Check sheet for the modelled part. Datum: model origin and axes. Units: mm. A direction names the side the tool comes from. Coordinates: 2 decimals unless noted, no trailing zeros. Loops run counter-clockwise (first coordinate to the right, second up) from the corner with the lowest first, then second, coordinate; pieces in that order, holes last.
```python
from build123d import *

# Parameters (mm, degrees)
SKETCH1_R                = 47.5
BOSS_EXTRUDE1_DEPTH      = 6
BOSS_EXTRUDE1_DEPTH_BACK = 6
SKETCH2_R                = 45
BOSS_EXTRUDE2_DEPTH      = 1
SKETCH3_R                = 45
BOSS_EXTRUDE3_DEPTH      = 1
SKETCH4_R                = 9
BOSS_EXTRUDE4_DEPTH      = 0.2
SKETCH5_R                = 9
BOSS_EXTRUDE5_DEPTH      = 5
SKETCH6_R                = 41
SKETCH6_R_2              = 9
CUT_EXTRUDE1_DEPTH       = 3
SKETCH7_R                = 41
SKETCH7_R_2              = 9
CUT_EXTRUDE2_DEPTH       = 3
SKETCH8_R                = 9
CUT_EXTRUDE3_DEPTH       = 17
SKETCH9_R                = 4
CUT_EXTRUDE4_DEPTH       = 20.2
CUT_EXTRUDE5_REACH       = 58.5
SKETCH10_R               = 1.6
CUT_EXTRUDE6_REACH       = 58.5
SKETCH11_R               = 1.6


with BuildPart() as part:
    # Sketch1 → Boss-Extrude1 (new body, two sides)
    with BuildSketch(Plane.XY) as boss_extrude1_sk:
        Circle(SKETCH1_R)
    extrude(amount=BOSS_EXTRUDE1_DEPTH)
    extrude(boss_extrude1_sk.sketch, amount=-BOSS_EXTRUDE1_DEPTH_BACK)

    # Sketch2 → Boss-Extrude2 (add)
    with BuildSketch(Plane.XY.offset(6)):
        Circle(SKETCH2_R)
    extrude(amount=BOSS_EXTRUDE2_DEPTH)

    # Sketch3 → Boss-Extrude3 (add)
    with BuildSketch(Plane(origin=(0, 0, -6), x_dir=(-1, 0, 0), z_dir=(0, 0, -1))):
        Circle(SKETCH3_R)
    extrude(amount=BOSS_EXTRUDE3_DEPTH)

    # Sketch4 → Boss-Extrude4 (add)
    with BuildSketch(Plane(origin=(0, 0, -7), x_dir=(-1, 0, 0), z_dir=(0, 0, -1))):
        Circle(SKETCH4_R)
    extrude(amount=BOSS_EXTRUDE4_DEPTH)

    # Sketch5 → Boss-Extrude5 (add)
    with BuildSketch(Plane.XY.offset(7)):
        Circle(SKETCH5_R)
    extrude(amount=BOSS_EXTRUDE5_DEPTH)

    # Sketch6 → Cut-Extrude1 (cut)
    with BuildSketch(Plane.XY.offset(7)):
        Circle(SKETCH6_R)
        Circle(SKETCH6_R_2, mode=Mode.SUBTRACT)
    extrude(amount=-CUT_EXTRUDE1_DEPTH, mode=Mode.SUBTRACT)

    # Sketch7 → Cut-Extrude2 (cut)
    with BuildSketch(Plane(origin=(0, 0, -7), x_dir=(-1, 0, 0), z_dir=(0, 0, -1))):
        Circle(SKETCH7_R)
        Circle(SKETCH7_R_2, mode=Mode.SUBTRACT)
    extrude(amount=-CUT_EXTRUDE2_DEPTH, mode=Mode.SUBTRACT)

    # Sketch8 → Cut-Extrude3 (cut, through all)
    with BuildSketch(Plane(origin=(0, 0, -4), x_dir=(-1, 0, 0), z_dir=(0, 0, -1))):
        with Locations((0, 25)):
            Circle(SKETCH8_R)
        with Locations((23.776412907, 7.725424859)):
            Circle(SKETCH8_R)
        with Locations((14.694631307, -20.225424859)):
            Circle(SKETCH8_R)
        with Locations((-14.694631307, -20.225424859)):
            Circle(SKETCH8_R)
        with Locations((-23.776412907, 7.725424859)):
            Circle(SKETCH8_R)
    extrude(amount=-CUT_EXTRUDE3_DEPTH, mode=Mode.SUBTRACT)

    # Sketch9 → Cut-Extrude4 (cut, through all)
    with BuildSketch(Plane.XY.offset(12)):
        Circle(SKETCH9_R)
    extrude(amount=-CUT_EXTRUDE4_DEPTH, mode=Mode.SUBTRACT)

    # Sketch10 → Cut-Extrude5 (cut, up to next)
    with BuildSketch(Plane.ZY.offset(9), mode=Mode.PRIVATE) as cut_extrude5_sk1:
        with Locations((8, 0)):
            Circle(SKETCH10_R)
    cut_extrude5_tool1 = extrude(cut_extrude5_sk1.sketch, amount=-CUT_EXTRUDE5_REACH, mode=Mode.PRIVATE) & part.part
    add(cut_extrude5_tool1.solids().sort_by_distance((-9, 0, 8))[0], mode=Mode.SUBTRACT)

    # Sketch11 → Cut-Extrude6 (cut, up to next)
    with BuildSketch(Plane(origin=(0, 9, 0), x_dir=(1, 0, 0), z_dir=(0, 1, 0)), mode=Mode.PRIVATE) as cut_extrude6_sk1:
        with Locations((0, -8)):
            Circle(SKETCH11_R)
    cut_extrude6_tool1 = extrude(cut_extrude6_sk1.sketch, amount=-CUT_EXTRUDE6_REACH, mode=Mode.PRIVATE) & part.part
    add(cut_extrude6_tool1.solids().sort_by_distance((0, 9, 8))[0], mode=Mode.SUBTRACT)


solid = part.part
```
1) Set-up check for faces 1 (the cylindrical face through (8.314, -3.447, 8.056)), 2 (the flat face through (-4, -2, -7.2)), 3 (the cylindrical face through (1.172, 8.923, -5.622)), 4 (the cylindrical face through (-0.35, 6.37, 9.56)), 5 (the cylindrical face through (1.846, -3.549, 2.534)): record each of +Z, -Z, +X, -X, +Y, -Y from which the full face is reachable in a straight line by a thin tool's end or side.
Answer sheet:
face 1: +Z
face 2: -Z, +X, -X, +Y, -Y
face 3: -Z
face 4: none
face 5: +Z, -Z
2) Section check B-B on y = 25. Enter the section's corners in (x, z), plus the area to 3 significant figures.
Answer sheet:
outline: (-40.39, -6) - (-37.42, -6) - (-37.42, -7) - (-32.5, -7) - (-32.5, -4) - (-9, -4) - (-9, 4) - (-32.5, 4) - (-32.5, 7) - (-37.42, 7) - (-37.42, 6) - (-40.39, 6) - close; (9, -4) - (32.5, -4) - (32.5, -7) - (37.42, -7) - (37.42, -6) - (40.39, -6) - (40.39, 6) - (37.42, 6) - (37.42, 7) - (32.5, 7) - (32.5, 4) - (9, 4) - close
area: 585 mm2
3) Section check D-D on y = 0. Give the number of separate pieces and of enclosed holes in the cut face, plus the area to 3 significant figures.
Answer sheet:
separate pieces: 5
enclosed holes: 0
area: 712 mm2
4) Section check C-C on z = -1.75. Enter the section's corners in (x, y).
Answer sheet:
outline: circle Ø95 at (0, 0); hole circle Ø18 at (-23.78, 7.73); hole circle Ø18 at (-14.69, -20.23); hole circle Ø18 at (0, 25); hole circle Ø8 at (0, 0); hole circle Ø18 at (14.69, -20.23); hole circle Ø18 at (23.78, 7.73)
5) Section check A-A on x = 21.5. Enter the section's corners in (y, z), plus the area to 3 significant figures.
Answer sheet:
outline: (-42.36, -6) - (-39.53, -6) - (-39.53, -7) - (-34.91, -7) - (-34.91, -4) - (-26.11, -4) - (-26.11, 4) - (-34.91, 4) - (-34.91, 7) - (-39.53, 7) - (-39.53, 6) - (-42.36, 6) - close; (-14.34, -4) - (-0.98, -4) - (-0.98, 4) - (-14.34, 4) - close; (16.43, -4) - (34.91, -4) - (34.91, -7) - (39.53, -7) - (39.53, -6) - (42.36, -6) - (42.36, 6) - (39.53, 6) - (39.53, 7) - (34.91, 7) - (34.91, 4) - (16.43, 4) - close
area: 522 mm2
6) Mould release check, pull along Z, two halves, no side actions. Record for faces 6 (the cylindrical face through (-6.37, 0.07, 6.4)), 7 (the flat face through (-10, -40, 7)), 8 (the cylindrical face through (6.11, -17.52, -0.06)): +Z half, -Z half, draft (parallel to the pull), parting line (faces both ways), or undercut.
Answer sheet:
face 6: undercut
face 7: +Z half
face 8: draft
7) Scan lines: line 1 (Y direction, x = 0, z = -2.5); line 2 (X direction, y = 9, z = 1.5); line 3 (Z direction, x = 35, y = 11). Record each from-to range of solid material in increasing order.
Answer sheet:
line 1: y = -47.5 to -4, 4 to 16, 34 to 47.5
line 2: x = -46.64 to -32.69, -14.87 to 14.87, 32.69 to 46.64
line 3: z = -4 to 4
8) Depth check by flat-ended pin: pin 1 (5 mm diameter, centred on y = -27, z = 7.5, fed in from +X); pin 2 (3 mm diameter, centred on x = -24, z = 5.5, fed in from -Y); pin 3 (1.5 mm diameter, centred on y = -28.5, z = -1.5, fed in from -X). Enter the tip coordinate at first touch or a pass-through.
Answer sheet:
pin 1: stops at x = 40.39
pin 2: stops at y = -41.83
pin 3: stops at x = -38.55
